```python
from build123d import *

# Parameters (mm, degrees)
BOSS_EXTRUDE1_START = -197
SKETCH1_R           = 1.5
BOSS_EXTRUDE1_DEPTH = 217
BOSS_EXTRUDE2_START = -4
BOSS_EXTRUDE2_DEPTH = 8


with BuildPart() as part:
    # Sketch1 → Boss-Extrude1 (new body)
    with BuildSketch(Plane(origin=(0, 0, 0), x_dir=(0, 0, -1), z_dir=(1, 0, 0)).offset(BOSS_EXTRUDE1_START)):
        Circle(SKETCH1_R)
    extrude(amount=BOSS_EXTRUDE1_DEPTH)

    # Sketch2 → Boss-Extrude2 (add)
    with BuildSketch(Plane.XY.offset(BOSS_EXTRUDE2_START)):
        Polygon((-10.858638704, -0.512581287), (-9.141361296, 0.512581287), (10.558638704, -32.487418713), (8.841361296, -33.512581287), align=None)
    extrude(amount=BOSS_EXTRUDE2_DEPTH)


solid = part.part
```
Check sheet for the modelled part. Datum: model origin and axes. Units: mm. Round coordinates to 2 decimals unless told otherwise and drop trailing zeros. Loops run counter-clockwise (first coordinate to the right, second up) from the corner with the lowest first, then second, coordinate; pieces in that order, holes last. Notation, with made-up numbers: (53.5, 1.25) -> (88.5, 1.25) arc R21 ccw to (88.5, 16.25) -> close; hole circle Ø3 at (-29, 74.25). An arc over 180 degrees is marked (long way). Answer in a Markdown table with one row per item.
Q1. Sectioned sample at A-A on x = 2. Enter the section's corners in (y, z).
Data:
| item | result |
|---|---|
| outline | (-22.05, -4) -> (-18.15, -4) -> (-18.15, 4) -> (-22.05, 4) -> close; circle Ø3 at (0, 0) |
Q2. Release check for a two-part mould opening along Y. For faces 1 (the face through (0, -16, -4)), 2 (the face through (0.571, -15.756, -0.056)), 3 (the face through (-0.871, -17.244, -0.056)) record: released by +Y, released by -Y, zero draft, split by the parting line, or undercut.
Data:
| item | result |
|---|---|
| face 1 | zero draft |
| face 2 | undercut |
| face 3 | released by -Y |
Q3. Sectioned sample at B-B on x = -162. Enter the section's corners in (y, z).
Data:
| item | result |
|---|---|
| outline | circle Ø3 at (0, 0) |
Q4. Sectioned sample at C-C on z = 2.75. Enter the section's corners in (x, y).
Data:
| item | result |
|---|---|
| outline | (-10.86, -0.51) -> (8.84, -33.51) -> (10.56, -32.49) -> (-9.14, 0.51) -> close |
Q5. Go/stop test with flat-tipped pins: P1, Ø3, axis at x = -77, z = -1.5, coming from the -Y side; P2, Ø3, axis at y = -22.5, z = 2.5, coming from the +X side; P3, Ø2, axis at y = -28, z = 1.5, coming from the +X side. Record where each tip stops, or that it passes through.
Data:
| item | result |
|---|---|
| P1 | stops at y = -1.5 |
| P2 | stops at x = 5.49 |
| P3 | stops at x = 8.48 |
Q6. Thickness scan on L1, parallel to Y at x = -124, z = 0.5; L2, parallel to X at y = -1.5, z = 3.25; L3, parallel to X at y = -26.5, z = 1. Record the ranges inside material, lowest first.
Data:
| item | result |
|---|---|
| L1 | y = -1.41 to 1.41 |
| L2 | x = -10.27 to -7.94 |
| L3 | x = 4.66 to 6.98 |
Q7. Sectioned sample at D-D on y = -18. Enter the section's corners in (x, z), then the cut area to 3 significant figures.
Data:
| item | result |
|---|---|
| outline | (-0.42, -4) -> (1.91, -4) -> (1.91, 4) -> (-0.42, 4) -> close |
| area | 18.6 mm^2 |
